from build123d import *

# Parameters (mm, degrees)
SKETCH1_R           = 6.5
BOSS_EXTRUDE1_DEPTH = 4
SKETCH2_R           = 2
CUT_EXTRUDE1_DEPTH  = 5
SKETCH4_R           = 1


with BuildPart() as part:
    # Sketch1 → Boss-Extrude1 (new body)
    with BuildSketch(Plane.XY):
        Circle(SKETCH1_R)
    extrude(amount=BOSS_EXTRUDE1_DEPTH)

    # Sketch2 → Cut-Extrude1 (cut, through all)
    with BuildSketch(Plane.XY.offset(4)):
        Circle(SKETCH2_R)
    extrude(amount=-CUT_EXTRUDE1_DEPTH, mode=Mode.SUBTRACT)

    # Cut-Sweep1: sweep along a path in Sketch3
    with BuildLine(Plane.XY.offset(2)) as cut_sweep1_path:
        CenterArc((0, 0), 6.5, 0, 360)
    # Sketch4 → Cut-Sweep1 (sweep, cut)
    with BuildSketch(Plane(origin=(0, 0, 0), x_dir=(0, 0, -1), z_dir=(1, 0, 0))):
        with Locations((-2, 6.5)):
            Circle(SKETCH4_R)
    sweep(path=cut_sweep1_path.line, mode=Mode.SUBTRACT)


solid = part.part
Verification items for the finished model (mm, model axes). Coordinates: 2 decimals unless noted, no trailing zeros. Order: outer loops, then holes, each group sorted by start corner. A loop starts at its lowest first (then second) coordinate and runs counter-clockwise, first axis right, second up.
Item 1: Section check C-C, the plane z = 2.6. Enter the section's corners in (x, y).
Filled in:
outline: circle Ø11.4 at (0, 0); hole circle Ø4 at (0, 0)
Item 2: Section check D-D, the plane z = 3.75. Enter the section's corners in (x, y), then the cut area to 3 significant figures.
Filled in:
outline: circle Ø13 at (0, 0); hole circle Ø4 at (0, 0)
area: 120 mm2
Item 3: Section check A-A, the plane x = 0. Enter the section's corners in (y, z), then the cut area to 3 significant figures.
Filled in:
outline: (-6.5, 0) - (-2, 0) - (-2, 4) - (-6.5, 4) - (-6.5, 3) arc R1 cw to (-6.5, 1) - close; (2, 0) - (6.5, 0) - (6.5, 1) arc R1 cw to (6.5, 3) - (6.5, 4) - (2, 4) - close
area: 32.9 mm2
Item 4: Material ranges on L1, parallel to Y at x = 0, z = 0.85; L2, parallel to X at y = -0.75, z = 0.95; L3, parallel to Z at x = 5.5, y = -3, recorded low to high.
Filled in:
L1: y = -6.5 to -2, 2 to 6.5
L2: x = -6.46 to -1.85, 1.85 to 6.46
L3: z = 0 to 1.03, 2.97 to 4
Item 5: Release check for a two-part mould opening along Y. For faces 1 (the face through (0, -2, 2)), 2 (the face through (-5.158, -3.955, 3.493)), 3 (the face through (1, 2, 0)) record: +Y half, -Y half, draft (parallel to the pull), parting line (faces both ways), or undercut.
Filled in:
face 1: undercut
face 2: parting line
face 3: draft
Item 6: Depth check by flat-ended pin: pin 1 (4 mm diameter, centred on x = 0.5, y = 0, fed in from -Z); pin 2 (2 mm diameter, centred on x = -2, z = 1.5, fed in from -Y). Enter the tip coordinate at first touch or a pass-through.
Filled in:
pin 1: stops at z = 0
pin 2: stops at y = -6.4
